Geometry check sheet. Reference: the model listing, model coordinates, mm. Give positions to 0.01 mm unless a question says otherwise; leave off trailing zeros. Order: outer loops, then holes, each group sorted by start corner. A loop starts at its lowest first (then second) coordinate and runs counter-clockwise, first axis right, second up. Notation, with made-up numbers: M -4,31.5 L 36,31.5 A9 cw 36,43.5 Z; hole C 20.5,71.5 d2. An arc over 180 degrees is marked long. Answer as CSV lines item,"result".
from build123d import *

# Parameters (mm, degrees)
SKETCH2_W           = 60
SKETCH2_H           = 10
BOSS_EXTRUDE1_DEPTH = 13
CUT_EXTRUDE1_DEPTH  = 3
SKETCH4_R           = 1.3
CUT_EXTRUDE2_DEPTH  = 33.015621187
FILLET1_R           = 3
FILLET2_R           = 3
SKETCH5_R           = 1.3
CUT_EXTRUDE3_DEPTH  = 10
SKETCH6_W           = 2
SKETCH6_H           = 5
CUT_EXTRUDE4_DEPTH  = 35.190641995


with BuildPart() as part:
    # Sketch2 → Boss-Extrude1 (new body)
    with BuildSketch(Plane.XY):
        Rectangle(SKETCH2_W, SKETCH2_H)
    extrude(amount=BOSS_EXTRUDE1_DEPTH)

    # Sketch3 → Cut-Extrude1 (cut)
    with BuildSketch(Plane(origin=(0, 0, 0), x_dir=(-1, 0, 0), z_dir=(0, 0, -1))):
        Polygon((-15, -3), (-12.401923789, -1.5), (-12.401923789, 1.5), (-15, 3), (-17.598076211, 1.5), (-17.598076211, -1.5), align=None)
        Polygon((15, -3), (17.598076211, -1.5), (17.598076211, 1.5), (15, 3), (12.401923789, 1.5), (12.401923789, -1.5), align=None)
    extrude(amount=-CUT_EXTRUDE1_DEPTH, mode=Mode.SUBTRACT)

    # Sketch4 → Cut-Extrude2 (cut, through all)
    with BuildSketch(Plane(origin=(0, 0, 3), x_dir=(-1, 0, 0), z_dir=(0, 0, -1))):
        with Locations((-15, 0)):
            Circle(SKETCH4_R)
        with Locations((15, 0)):
            Circle(SKETCH4_R)
    extrude(amount=-CUT_EXTRUDE2_DEPTH, mode=Mode.SUBTRACT)

    # Fillet1
    # the kernel refuses this fillet: 3 mm, written as the material it takes off along each edge
    with BuildSketch(Plane(origin=(37.5, -5, 0), x_dir=(0, 1, 0), z_dir=(-1, 0, 0))) as fillet1_piece_1:
        with BuildLine():
            CenterArc((FILLET1_R, -FILLET1_R), FILLET1_R, 90, 90)
            Line((0, -FILLET1_R), (0, 0))
            Line((0, 0), (FILLET1_R, 0))
        make_face()
    extrude(amount=75, mode=Mode.SUBTRACT)
    with BuildSketch(Plane(origin=(-37.5, 5, 0), x_dir=(0, 0, 1), z_dir=(1, 0, 0))) as fillet1_piece_2:
        with BuildLine():
            CenterArc((FILLET1_R, FILLET1_R), FILLET1_R, 180, 90)
            Line((0, FILLET1_R), (0, 0))
            Line((0, 0), (FILLET1_R, 0))
        make_face()
    extrude(amount=75, mode=Mode.SUBTRACT)

    # Fillet2
    fillet2_edges = [part.edges().sort_by_distance(p)[0] for p in [
        (-30, 0, 13),
        (30, 0, 13),
    ]]
    fillet(fillet2_edges, radius=FILLET2_R)

    # Sketch5 → Cut-Extrude3 (cut)
    with BuildSketch(Plane(origin=(30, 0, 0), x_dir=(0, 0, -1), z_dir=(1, 0, 0))):
        with Locations(Location((-6, 0, 0), (0, 0, 90))):
            Circle(SKETCH5_R)
    cut_extrude3 = extrude(amount=-CUT_EXTRUDE3_DEPTH, mode=Mode.SUBTRACT)

    # Sketch6 → Cut-Extrude4 (cut, symmetric)
    with BuildSketch(Plane(origin=(0, 5, 0), x_dir=(1, 0, 0), z_dir=(0, 1, 0))):
        with Locations((20, -6)):
            Rectangle(SKETCH6_W, SKETCH6_H)
    cut_extrude4 = extrude(amount=CUT_EXTRUDE4_DEPTH, both=True, mode=Mode.SUBTRACT)

    # Mirror1: Cut-Extrude3, Cut-Extrude4 across plane
    add(cut_extrude3.mirror(Plane(origin=(0, 0, 0), x_dir=(0, 0, 1), z_dir=(1, 0, 0))), mode=Mode.SUBTRACT)
    add(cut_extrude4.mirror(Plane(origin=(0, 0, 0), x_dir=(0, 0, 1), z_dir=(1, 0, 0))), mode=Mode.SUBTRACT)


solid = part.part
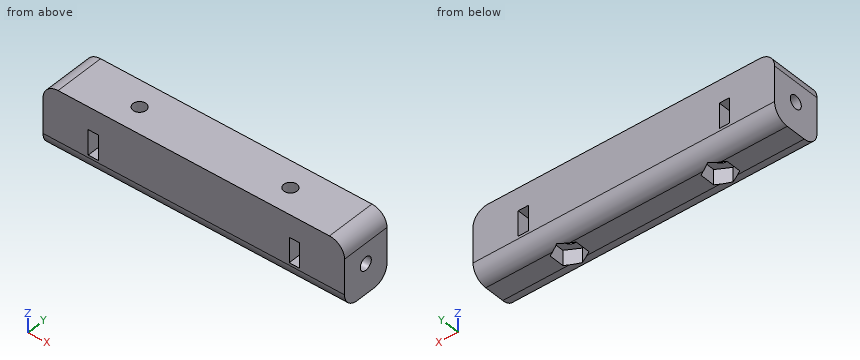
(1) Section check B-B on x = -26. Enter the section's corners in (y, z).
The answers:
outline,"M -5,3 A3 ccw -2,0 L 2,0 A3 ccw 5,3 L 5,13 L -5,13 Z; hole C 0,6 d2.6"
(2) Section check C-C on x = -14.5. Enter the section's corners in (y, z).
The answers:
outline,"M -5,3 A3 ccw -2.71,0.09 L -2.71,3 L -1.2,3 L -1.2,13 L -5,13 Z; M 1.2,3 L 2.71,3 L 2.71,0.09 A3 ccw 5,3 L 5,13 L 1.2,13 Z"
(3) Section check A-A on z = 4. Enter the section's corners in (x, y).
The answers:
outline,"M -30,-5 L -21,-5 L -21,5 L -30,5 Z; M -19,-5 L 19,-5 L 19,5 L -19,5 Z; M 21,-5 L 30,-5 L 30,5 L 21,5 Z; hole C -15,0 d2.6; hole C 15,0 d2.6"
(4) Material ranges on line 1 (Z direction, x = 26, y = 0); line 2 (X direction, y = 3, z = 3.75); line 3 (X direction, y = 2.25, z = 1.25), recorded low to high.
The answers:
line 1,"z = 0 to 4.7, 7.3 to 13"
line 2,"x = -30 to -21, -19 to 19, 21 to 30"
line 3,"x = -30 to -16.3, -13.7 to 13.7, 16.3 to 30"
(5) Gauge pin test, flat ends, axial feed: P1, Ø0.6, axis at x = -19.5, y = -2.5, coming from the -Z side; P2, Ø2.5, axis at x = -15, y = 0, coming from the +Z side; P3, Ø2.5, axis at y = 0, z = 6, coming from the -X side. Record the tip position at first contact, or that the pin passes through.
The answers:
P1,"stops at z = 0.01"
P2,"passes through"
P3,"stops at x = -19"
(6) Section check D-D on y = 0. State how many separate pieces and enclosed holes the cut face has, then the cut area to 3 significant figures.
The answers:
separate pieces,"3"
enclosed holes,"0"
area,"626 mm2"
